Autodesk Inventor part; units mm, degrees
ref_plane "YZ Plane" through (0, 0, 0) normal (1, 0, 0) x (0, 1, 0)
ref_plane "XZ Plane" through (0, 0, 0) normal (0, 1, 0) x (-1, 0, 0)
ref_plane "XY Plane" through (0, 0, 0) normal (0, 0, 1) x (1, 0, 0)
sketch "Sketch1" plane through (0, 0, 0) normal (0, 0, 1) x (1, 0, 0)
  line L0 (150, -100) -> (150, 100)
  line L1 (-150, -100) -> (150, -100)
  line L2 (150, 100) -> (-150, 100)
  line L3 (-150, 100) -> (-150, -100)
  line L4 (0, 100) -> (0, 0) construction
  line L5 (0, 0) -> (0, -100) construction
  line L6 (0, -50) -> (150, -50) construction
  line L7 (0, 50) -> (150, 50) construction
  line L8 (0, 50) -> (-150, 50) construction
  line L9 (0, -50) -> (-150, -50) construction
  line L10 (-150, -50) -> (-158.805, -50) construction
  circle A0 centre (-158.805, -50) radius 8.805
  circle A1 centre (-158.805, -50) radius 2.805
  circle A2 centre (-158.805, 50) radius 2.805
  circle A3 centre (-158.805, 50) radius 8.805
  line L11 (150, -50) -> (158.805, -50) construction
  circle A4 centre (158.805, -50) radius 8.805
  circle A5 centre (158.805, -50) radius 2.805
  circle A6 centre (158.805, 50) radius 8.805
  circle A7 centre (158.805, 50) radius 2.805
  line L12 (158.805, 41.195) -> (150, 41.195)
  line L13 (158.805, 58.805) -> (150, 58.805)
  line L14 (158.805, -41.195) -> (150, -41.195)
  line L15 (158.805, -58.805) -> (150, -58.805)
  line L16 (-158.805, -58.805) -> (-150, -58.805)
  line L17 (-158.805, -41.195) -> (-150, -41.195)
  line L18 (-158.805, 41.195) -> (-150, 41.195)
  line L19 (-158.805, 58.805) -> (-150, 58.805)
  dimension "d0" = 8.805
  dimension "d1" = 5.61
  dimension "d2" = 5.61
  dimension "d3" = 8.805
  dimension "d4" = 5.61
extrude "Plate1" add sketch "Sketch1" along normal blind 6
fillet "Corner Round1" radius 3.175 8 edges at (-150, -58.805, 3) (-150, -41.195, 3) (-150, 41.195, 3) (-150, 58.805, 3) (150, 58.805, 3) (150, 41.195, 3) (150, -41.195, 3) (150, -58.805, 3)
equation "\"d7\" = Thickness"
equation "\"BendRadius\" = Thickness"
equation "\"BendReliefWidth\" = Thickness"
equation "\"BendReliefDepth\" = 0.5 * Thickness"
equation "\"CornerReliefSize\" = 4 * Thickness"
equation "\"MinimumRemnant\" = 2 * Thickness"
equation "\"TransitionRadius\" = BendRadius"
equation "\"JacobiRadiusSize\" = BendRadius"
equation "\"GapSize\" = Thickness"
properties part number "bed-plate"
Check sheet for the modelled part. Datum: model origin and axes. Units: mm. A direction names the side the tool comes from. Round coordinates to 2 decimals unless told otherwise and drop trailing zeros. Order: outer loops, then holes, each group sorted by start corner. A loop starts at its lowest first (then second) coordinate and runs counter-clockwise, first axis right, second up.
(1) Scan lines: probe 1 along X at (y, z) = (-51, 1.6); probe 2 along X at (y, z) = (-72.5, 2). Record each from-to range of solid material in increasing order.
(2) Draft check along Y on faces 1 (the flat face through (2, 100, 3)), 2 (the flat face through (150, 81, 3)), 3 (the cylindrical face through (167.608, -49.806, 2.958)). Enter one of: pulls with the +Y half, pulls with the -Y half, needs draft (parallel to the pull), parting line crosses it, or undercut.
(3) Go/stop test with flat-tipped pins: P1, Ø1.7, axis at x = -156, z = 4, coming from the +Y side (3 decimals); P2, Ø1.7, axis at x = 156, z = 4, coming from the -Y side (3 decimals); P3, Ø1.5, axis at y = 53, z = 3, coming from the -X side; P4, Ø4.5, axis at x = -158.805, y = -50, coming from the +Z side. Record where each tip stops, or that it passes through.
(4) Cross-section at B-B, the plane y = 79. Enter the section's corners in (x, z).
(5) Access from +Z, -Z, +X, -X, +Y, -Y to the whole of each face (thin tool, end or side, straight path). Record for faces 4 (the flat face through (-150, 1, 3)), 5 (the flat face through (-150, -81, 3)), 6 (the flat face through (150, -1, 3)), 7 (the flat face through (-150, 81, 3)), 8 (the flat face through (150, -81, 3)).
(6) Cross-section at A-A, the plane z = 2.6. State how many separate pieces and enclosed holes the cut face has, and give its area (3 significant figures).
Check sheet entries:
1. probe 1: x = -167.55 to -161.43, -156.18 to 156.18, 161.43 to 167.55
1. probe 2: x = -150 to 150
2. face 1: pulls with the +Y half
2. face 2: needs draft
2. face 3: undercut
3. P1: stops at y = 58.805
3. P2: stops at y = -58.805
3. P3: stops at x = -167.32
3. P4: passes through
4. outline: (-150, 0) - (150, 0) - (150, 6) - (-150, 6) - close
5. face 4: +Z, -Z, -X
5. face 5: +Z, -Z, -X, -Y
5. face 6: +Z, -Z, +X
5. face 7: +Z, -Z, -X, +Y
5. face 8: +Z, -Z, +X, -Y
6. separate pieces: 1
6. enclosed holes: 4
6. area: 61,000 mm2
